Input: part model. Units: mm. Frame: model coordinates. A direction names the side the tool comes from. Give positions to 0.01 mm unless a question says otherwise; leave off trailing zeros. Loops run counter-clockwise (first coordinate to the right, second up) from the corner with the lowest first, then second, coordinate; pieces in that order, holes last. Notation, with made-up numbers: (82, -37.75) - (101, -37.75) arc R10 cw to (101, -30.75) - close; hole circle Ø7 at (46.5, 37). An arc over 180 degrees is marked (long way). One line per item, written item: value.
from build123d import *

# Parameters (mm, degrees)
F0_R      = 2
F1_DEPTH  = 56
F0_R_2    = 3.0739118257
F1_FACE_R = 2
F2_DEPTH  = 2
F3_R      = 2


with BuildPart() as f1:
    # F0 (on Top) → F1 (new body)
    with BuildSketch(Plane.XY):
        Circle(F0_R)
    extrude(amount=F1_DEPTH)

    # F0 (on Top) + F1_face (on face) → F2 (join)
    with BuildSketch(Plane.XY):
        Circle(F0_R_2)
        Circle(F0_R, mode=Mode.SUBTRACT)
    with BuildSketch(Plane(origin=(0, 0, 0), x_dir=(1, 0, 0), z_dir=(0, 0, -1))):
        Circle(F1_FACE_R)
    extrude(amount=F2_DEPTH, dir=(0, 0, 1))

    # F3
    f3_edges = [f1.edges().sort_by_distance(p)[0] for p in [
        (-2, 0, 56),
    ]]
    fillet(f3_edges, radius=F3_R)


solid = f1.part
Item 1: Section C-C, the plane z = 31. Output: boundary loops of the cut face in (x, y).
Verdict:
outline: circle Ø4 at (0, 0)
Item 2: Access query for faces 1 (the face through (2.932, 0.923, 0.986)), 2 (the face through (0, -2, 28)). Directions: +Z, -Z, +X, -X, +Y, -Y. A direction counts if a zero-diameter tool reaches every point of the face in a straight line with its end or side. Return the directions, or none.
Verdict:
face 1: +Z, -Z
face 2: +Z
Item 3: Section A-A, the plane y = 0. Output: boundary loops of the cut face in (x, z).
Verdict:
outline: (-3.07, 0) - (3.07, 0) - (3.07, 2) - (2, 2) - (2, 54) arc R2 ccw to (-2, 54) - (-2, 2) - (-3.07, 2) - close
Item 4: Material intervals for L1, parallel to Z at x = 0.75, y = -2.5; L2, parallel to Z at x = -0.25, y = 0; L3, parallel to X at y = -0.75, z = 46.5, sorted ascending.
Verdict:
L1: z = 0 to 2
L2: z = 0 to 55.98
L3: x = -1.85 to 1.85
Item 5: Pin query (flat end, axial travel): P1, Ø3, axis at y = -1.5, z = 32.5, coming from the -X side; P2, Ø2, axis at y = 2, z = 17, coming from the +X side; P3, Ø1.5, axis at y = -2.5, z = 13.5, coming from the +X side. Return the tip coordinate at first contact, or that it passes through.
Verdict:
P1: stops at x = -2
P2: stops at x = 1.73
P3: stops at x = 0.97
Item 6: Section D-D, the plane x = -2.5. Output: boundary loops of the cut face in (y, z), and give its area (3 significant figures).
Verdict:
outline: (-1.79, 0) - (1.79, 0) - (1.79, 2) - (-1.79, 2) - close
area: 7.15 mm^2
